The model under review builds one solid part; all positions refer to its coordinate system, in mm. Face numbers are marked on the shaded views. A direction names the side the tool comes from. Round coordinates to 2 decimals unless told otherwise and drop trailing zeros. Write each loop counter-clockwise with the first axis right and the second up, starting at its lowest first coordinate (ties: lowest second). Pieces come first, ordered by that corner, then holes. Notation, with made-up numbers: (4, -34) -> (54, -34) arc R27 cw to (54, -3) -> close; hole circle Ø2 at (32, 67). An arc over 180 degrees is marked (long way). Answer as a JSON object with one key per item and string values. Group by question number.
1) We need section A-A, the plane x = 0. Write out the cut boundary in (y, z), then the cut area to 3 significant figures.
2) Machinability: for the marked faces 5, 6, 7, 8 and 9, which of the approach directions +Z, -Z, +X, -X, +Y, -Y give a long, thin tool a straight path to every point of the face, cutting with its end or side? Answer none if there is none.
3) To check wall thickness, follow probe 1 along Z at (x, y) = (-54, 154); probe 2 along X at (y, z) = (156.25, -61); probe 3 along Z at (x, y) = (14.5, 186). State the ranges of each line that lie inside material, in increasing order. Write a range as [from, to].
4) We need section D-D, the plane y = 195.5. Write out the cut boundary in (x, z).
5) Insertion check: pin 1 Ø17.5 at (y, z) = (204, -33) entering from +X; pin 2 Ø24 at (y, z) = (210.5, -33.5) entering from -X; pin 3 Ø6.5 at (y, z) = (178, 34) entering from +X. Each pin has a flat end and moves straight along its axis. Give the tip position at first contact, or say it passes through.
6) We need section B-B, the plane z = -61. Write out the cut boundary in (x, y), then the cut area to 3 significant figures.
7) We need section C-C, the plane y = 213. Write out the cut boundary in (x, z), then the cut area to 3 significant figures.
8) Mouldability with a two-part tool opening along X and no side actions: class the marked faces 1, 2, 3 and 4 as pulls with the +X half, pulls with the -X half, needs draft (parallel to the pull), parting line crosses it, or undercut.
from build123d import *

# Parameters (mm, degrees)
SKETCH8_W                       = 140
SKETCH8_H                       = 10
BOSS_EXTRUDE6_DEPTH             = 77
BOSS_EXTRUDE6_2_DEPTH           = 77
SKETCH9_R                       = 6.5
CUT_EXTRUDE3_POS_1_2_DEPTH      = 160
CUT_EXTRUDE3_POS_1_2_DEPTH_BACK = 160
SKETCH3_R                       = 12.5
BOSS_EXTRUDE2_POS_1_2_DEPTH     = 22
SKETCH16_W                      = 251.646803711
SKETCH16_H                      = 83.728976974
CUT_EXTRUDE4_DEPTH              = 58
CUT_EXTRUDE4_DEPTH_BACK         = 98


with BuildPart() as part:
    # Sketch8 → Boss-Extrude6 (new body, symmetric)
    with BuildSketch(Plane.XY):
        with Locations((0, 155)):
            Rectangle(SKETCH8_W, SKETCH8_H)
    extrude(amount=BOSS_EXTRUDE6_DEPTH, both=True)


with BuildPart() as body_2:
    # Sketch8 → Boss-Extrude6 2 (new body, symmetric)
    with BuildSketch(Plane.XY):
        with Locations((0, -5)):
            Rectangle(SKETCH8_W, SKETCH8_H)
    extrude(amount=BOSS_EXTRUDE6_2_DEPTH, both=True)


with BuildPart() as cut_extrude3_pos_1_2_tool:
    # Sketch9 → Cut-Extrude3 _pos 1_2 (new body, two sides)
    with BuildSketch(Plane(origin=(0, 0, 0), x_dir=(1, 0, 0), z_dir=(0, 1, 0))) as cut_extrude3_pos_1_2_sk:
        with Locations((54, 61)):
            Circle(SKETCH9_R)
        with Locations((-54, 61)):
            Circle(SKETCH9_R)
        with Locations((-54, -61)):
            Circle(SKETCH9_R)
        with Locations((54, -61)):
            Circle(SKETCH9_R)
    extrude(amount=CUT_EXTRUDE3_POS_1_2_DEPTH)
    extrude(cut_extrude3_pos_1_2_sk.sketch, amount=-CUT_EXTRUDE3_POS_1_2_DEPTH_BACK)


with BuildPart() as part_1:
    add(part.part)

    # Cut-Extrude3 _pos 1_2: cut by cut_extrude3_pos_1_2_tool
    add(cut_extrude3_pos_1_2_tool.part, mode=Mode.SUBTRACT)

    # Sketch3 → Boss-Extrude2 _pos 1_2 (add)
    with BuildSketch(Plane.XY.offset(20)):
        with BuildLine():
            Line((55, 160), (55, 185))
            Line((55, 185), (28, 185))
            Line((28, 185), (28, 223))
            ThreePointArc((28, 223), (0, 251), (-28, 223))
            Line((-28, 223), (-28, 185))
            Line((-28, 185), (-55, 185))
            Line((-55, 185), (-55, 160))
            Line((-55, 160), (55, 160))
        make_face()
        with Locations((0, 223)):
            Circle(SKETCH3_R, mode=Mode.SUBTRACT)
    boss_extrude2_pos_1_2 = extrude(amount=BOSS_EXTRUDE2_POS_1_2_DEPTH)

    # Mirror4: Boss-Extrude2 _pos 1_2 across plane
    add(boss_extrude2_pos_1_2.mirror(Plane.XY))


with BuildPart() as body_2_1:
    add(body_2.part)

    # Cut-Extrude3 _pos 1_2: cut by cut_extrude3_pos_1_2_tool
    add(cut_extrude3_pos_1_2_tool.part, mode=Mode.SUBTRACT)

    # Sketch16 → Cut-Extrude4 (cut, two sides)
    with BuildSketch(Plane.XY.offset(20)) as cut_extrude4_sk:
        with Locations((-3.761561591, 8.391166305)):
            Rectangle(SKETCH16_W, SKETCH16_H)
    extrude(amount=CUT_EXTRUDE4_DEPTH, mode=Mode.SUBTRACT)
    extrude(cut_extrude4_sk.sketch, amount=-CUT_EXTRUDE4_DEPTH_BACK, mode=Mode.SUBTRACT)


solid = part_1.part
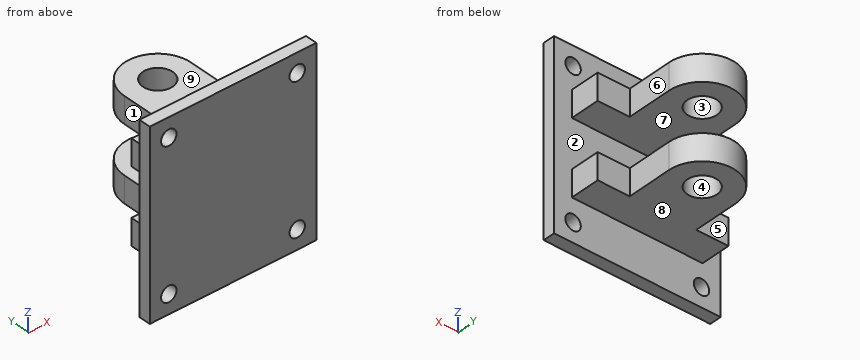
Here are the results:
{
 "1": {"outline": "(150, -77) -> (160, -77) -> (160, -42) -> (210.5, -42) -> (210.5, -20) -> (160, -20) -> (160, 20) -> (210.5, 20) -> (210.5, 42) -> (160, 42) -> (160, 77) -> (150, 77) -> close; (235.5, -42) -> (251, -42) -> (251, -20) -> (235.5, -20) -> close; (235.5, 20) -> (251, 20) -> (251, 42) -> (235.5, 42) -> close", "area": "4,440 mm^2"},
 "2": {"face 5": "+Z, -Z, -X, +Y", "face 6": "+Z, -Z, +X, +Y", "face 7": "+X, -X, +Y", "face 8": "-Z, +X, -X, +Y", "face 9": "+Z, +X, -X, +Y"},
 "3": {"probe 1": "z = [-77, -67.5], [-54.5, 54.5], [67.5, 77]", "probe 2": "x = [-70, -60.5], [-47.5, 47.5], [60.5, 70]", "probe 3": "z = [-42, -20], [20, 42]"},
 "4": {"outline": "(-28, -42) -> (28, -42) -> (28, -20) -> (-28, -20) -> close; (-28, 20) -> (28, 20) -> (28, 42) -> (-28, 42) -> close"},
 "5": {"pin 1": "stops at x = 28", "pin 2": "stops at x = -28", "pin 3": "stops at x = 55"},
 "6": {"outline": "(-70, 150) -> (-60.5, 150) -> (-60.5, 160) -> (-70, 160) -> close; (-47.5, 150) -> (47.5, 150) -> (47.5, 160) -> (-47.5, 160) -> close; (60.5, 150) -> (70, 150) -> (70, 160) -> (60.5, 160) -> close", "area": "1,140 mm^2"},
 "7": {"outline": "(-28, -42) -> (-7.5, -42) -> (-7.5, -20) -> (-28, -20) -> close; (-28, 20) -> (-7.5, 20) -> (-7.5, 42) -> (-28, 42) -> close; (7.5, -42) -> (28, -42) -> (28, -20) -> (7.5, -20) -> close; (7.5, 20) -> (28, 20) -> (28, 42) -> (7.5, 42) -> close", "area": "1,800 mm^2"},
 "8": {"face 1": "pulls with the -X half", "face 2": "needs draft", "face 3": "undercut", "face 4": "undercut"}
}
